```python
from build123d import *

# Parameters (mm, degrees)
BOSS_EXTRUDE1_DEPTH = 12.7
SHELL1_START        = -12.7
SHELL1_DEPTH        = 10.16
FILLET1_R           = 0.508
SKETCH2_R           = 6.35
SKETCH2_R_2         = 3.96875
BOSS_EXTRUDE2_DEPTH = 20.32
SKETCH3_R           = 3.96875
CUT_EXTRUDE1_DEPTH  = 31.743483417


# Read off the part's stored shape, not the designer's step: Shell1
with BuildPart() as part:
    # Sketch1 → Boss-Extrude1 (new body)
    with BuildSketch(Plane(origin=(0, 0, 0), x_dir=(1, 0, 0), z_dir=(0, 1, 0))):
        with BuildLine():
            Line((-21.893352199, -2.46416195), (-0.616040488, -7.783489878))
            ThreePointArc((-0.616040488, -7.783489878), (0, -7.859327928), (0.616040488, -7.783489878))
            Line((0.616040488, -7.783489878), (21.893352199, -2.46416195))
            ThreePointArc((21.893352199, -2.46416195), (23.817311711, 0), (21.893352199, 2.46416195))
            Line((21.893352199, 2.46416195), (0.616040488, 7.783489878))
            ThreePointArc((0.616040488, 7.783489878), (0, 7.859327928), (-0.616040488, 7.783489878))
            Line((-0.616040488, 7.783489878), (-21.893352199, 2.46416195))
            ThreePointArc((-21.893352199, 2.46416195), (-23.817311711, 0), (-21.893352199, -2.46416195))
        make_face()
    extrude(amount=-BOSS_EXTRUDE1_DEPTH)

    # Shell1 outline → Shell1 (cut)
    with BuildSketch(Plane(origin=(0, 0, 0), x_dir=(1, 0, 0), z_dir=(0, 1, 0)).offset(SHELL1_START)):
        Polygon((-21.277311711, 0), (0, -5.319327928), (21.277311711, 0), (0, 5.319327928), align=None)
    extrude(amount=SHELL1_DEPTH, mode=Mode.SUBTRACT)

    # Fillet1
    fillet1_edges = [part.edges().sort_by_distance(p)[0] for p in [
        (21.277311711, -7.62, 0),
        (0, -7.62, 5.319327928),
        (-21.277311711, -7.62, 0),
        (0, -7.62, -5.319327928),
    ]]
    fillet(fillet1_edges, radius=FILLET1_R)

    # Sketch2 → Boss-Extrude2 (add)
    with BuildSketch(Plane(origin=(0, 0, 0), x_dir=(1, 0, 0), z_dir=(0, 1, 0))):
        with Locations(Location((0, 0, 0), (0, 0, 270))):
            Circle(SKETCH2_R)
        with Locations(Location((0, 0, 0), (0, 0, 270))):
            Circle(SKETCH2_R_2, mode=Mode.SUBTRACT)
    extrude(amount=-BOSS_EXTRUDE2_DEPTH)

    # Sketch3 → Cut-Extrude1 (cut, through all)
    with BuildSketch(Plane.XZ.offset(2.54)):
        with Locations(Location((0, 0, 0), (0, 0, 90))):
            Circle(SKETCH3_R)
    extrude(amount=-CUT_EXTRUDE1_DEPTH, mode=Mode.SUBTRACT)


solid = part.part
```
Can you work these out from the model? Positions are in its coordinate system, mm. A direction names the side the tool comes from. Coordinates: 2 decimals unless noted, no trailing zeros. Loops run counter-clockwise (first coordinate to the right, second up) from the corner with the lowest first, then second, coordinate; pieces in that order, holes last. Notation, with made-up numbers: M 40.25,31.25 L 62.25,31.25 A27 cw 62.25,64.25 Z; hole C 9.5,-39 d7. An arc over 180 degrees is marked long. Put each result on its own line as item: value. Start each with the question number.
(1) Imagine slicing it at B-B on x = 0. List the corners of the cut face in (y, z) for me.
(2) Will these pins go through, and if not, where does the flat tip stop? pin 1 Ø1.5 at (x, y) = (5, -5.5) entering from -Z (3 decimals); pin 2 Ø3 at (x, y) = (12.5, -11) entering from -Z; pin 3 Ø2.5 at (x, z) = (14, -1.5) entering from -Y.
(3) Which directions (+Z, -Z, +X, -X, +Y, -Y) give clear straight access to the entire face, cutting with the end or side of a thin tool? Please do faces 4 (the face through (-0.01, -6.26, 7.86)), 5 (the face through (11, -2.54, 0)).
(4) Imagine slicing it at C-C on y = -14.75. List the corners of the cut face in (x, z) for me, and give its area (3 significant figures).
(5) Imagine slicing it at D-D on z = 2. List the corners of the cut face in (x, y) for me, and give its area (3 significant figures).
(6) Imagine slicing it at A-A on z = 0. List the corners of the cut face in (x, y) for me, and give its area (3 significant figures).
(7) I need wall thicknesses on probe 1 along X at (y, z) = (-8, 0); probe 2 along Z at (x, y) = (0, -13.75); probe 3 along Z at (x, y) = (0, -9.75). Which ranges of each line are inside material? Lowest first, please.
(8) We'd pull the mould along X, two halves only. Please class faces 1 (the face through (-19.69, -7.55, 0.01)), 2 (the face through (11.404, -6.261, -5.087)), 3 (the face through (-23.817, -6.261, -0.047)): +X half, -X half, draft (parallel to the pull), parting line (faces both ways), or undercut.
Worked answers:
1. outline: M -20.32,-6.35 L -12.7,-6.35 L -12.7,-7.86 L 0,-7.86 L 0,-3.97 L -20.32,-3.97 Z; M -20.32,3.97 L 0,3.97 L 0,7.86 L -12.7,7.86 L -12.7,6.35 L -20.32,6.35 Z
2. pin 1: stops at z = -6.875
2. pin 2: stops at z = -5.19
2. pin 3: stops at y = -12.7
3. face 4: +Z, +Y, -Y
3. face 5: -Y
4. outline: C 0,0 d12.7; hole C 0,0 d7.94
4. area: 77.2 mm2
5. outline: M -22.84,-12.7 L -13.28,-12.7 L -13.28,-2.54 L -6.03,-2.54 L -6.03,-20.32 L -3.43,-20.32 L -3.43,0 L -22.84,0 Z; M 3.43,-20.32 L 6.03,-20.32 L 6.03,-2.54 L 13.28,-2.54 L 13.28,-12.7 L 22.84,-12.7 L 22.84,0 L 3.43,0 Z
5. area: 385 mm2
6. outline: M -23.82,-12.7 L -19.69,-12.7 L -19.69,-2.54 L -6.35,-2.54 L -6.35,-20.32 L -3.97,-20.32 L -3.97,0 L -23.82,0 Z; M 3.97,-20.32 L 6.35,-20.32 L 6.35,-2.54 L 19.69,-2.54 L 19.69,-12.7 L 23.82,-12.7 L 23.82,0 L 3.97,0 Z
6. area: 269 mm2
7. probe 1: x = -23.82 to -19.69, -6.35 to -3.97, 3.97 to 6.35, 19.69 to 23.82
7. probe 2: z = -6.35 to -3.97, 3.97 to 6.35
7. probe 3: z = -7.86 to -3.97, 3.97 to 7.86
8. face 1: undercut
8. face 2: +X half
8. face 3: -X half
